Model file for the job. Use its own axes, mm. A direction names the side the tool comes from. Coordinates: 2 decimals unless noted, no trailing zeros. Order: outer loops, then holes, each group sorted by start corner. A loop starts at its lowest first (then second) coordinate and runs counter-clockwise, first axis right, second up. Notation, with made-up numbers: (-12, 13) - (8, 13) arc R27 cw to (8, 49) - close; hole circle Ø7 at (-21, 54). An arc over 180 degrees is marked (long way). Put each result on its own line as item: value. Start each with the question number.
Autodesk Fusion 360 part; units mm, degrees
sketch "Sketch1" plane through (0, 0, 0) normal (0, 0, 1) x (1, 0, 0)
  line L0 (0, 0) -> (60, 0)
  line L1 (60, 0) -> (60, -25)
  line L2 (60, -25) -> (0, -25)
  line L3 (0, -25) -> (0, 0)
  line L4 (5, -5) -> (55, -5)
  line L5 (55, -5) -> (55, -20)
  line L6 (55, -20) -> (5, -20)
  line L7 (5, -20) -> (5, -5)
  line L8 (41, -10.5) -> (45, -10.5)
  line L9 (45, -10.5) -> (45, -14.5)
  line L10 (45, -14.5) -> (41, -14.5)
  line L11 (41, -14.5) -> (41, -10.5)
  line L12 (15, -10.5) -> (19, -10.5)
  line L13 (19, -10.5) -> (19, -14.5)
  line L14 (19, -14.5) -> (15, -14.5)
  line L15 (15, -14.5) -> (15, -10.5)
  dimension "d1" = 60
  dimension "d2" = 25
  dimension "d3" = 50
  dimension "d4" = 15
  dimension "d5" = 5
  dimension "d6" = 5
  dimension "d7" = 4
  dimension "d8" = 10
  dimension "d9" = 5.5
  dimension "d10" = 4
  dimension "d11" = 4
  dimension "d12" = 5.5
  dimension "d13" = 10
  dimension "d14" = 4
extrude "Extrude1" add sketch "Sketch1" along normal blind 2 contours L0 L1 L2 L3
sketch "Sketch2" plane through (0, 0, 0) normal (0, 0, 1) x (1, 0, 0)
  line L0 (15, -10.5) -> (19, -10.5)
  line L1 (19, -10.5) -> (19, -14.5)
  line L2 (19, -14.5) -> (15, -14.5)
  line L3 (15, -14.5) -> (15, -10.5)
  line L4 (41, -10.5) -> (45, -10.5)
  line L5 (45, -10.5) -> (45, -14.5)
  line L6 (45, -14.5) -> (41, -14.5)
  line L7 (41, -14.5) -> (41, -10.5)
  line L8 (55, -5) -> (55, -20)
  line L9 (55, -20) -> (5, -20)
  line L10 (5, -20) -> (5, -5)
  line L11 (5, -5) -> (55, -5)
  dimension "d17" = 4
  dimension "d18" = 10
  dimension "d19" = 5.5
  dimension "d20" = 4
  dimension "d21" = 4
  dimension "d22" = 10
  dimension "d23" = 5.5
  dimension "d24" = 4
extrude "Extrude2" add sketch "Sketch2" along normal blind 5
extrude "Extrude3" add 1 faces at (40, -25, 0.6667) along direction (0, -1, 0) blind 10
extrude "Extrude4" add 1 faces at (20, 0, 0.6667) along direction (0, 1, 0) blind 10
sketch "Sketch3" plane through (0, -35, 0) normal (0, -1, 0) x (1, 0, 0)
  line L0 (0, 0) -> (60, 0)
  line L1 (60, 0) -> (60, 2)
  line L2 (60, 2) -> (0, 2)
  line L3 (0, 2) -> (0, 0)
  line L4 (25, 0) -> (35, 0)
  line L5 (35, 0) -> (35, 1)
  line L6 (35, 1) -> (25, 1)
  line L7 (25, 1) -> (25, 0)
  line L8 (41, 0) -> (41, 5)
  dimension "d31" = 1
  dimension "d32" = 6
  dimension "d33" = 10
extrude "Extrude5" add sketch "Sketch3" along normal blind 50 contours L0 L4 L5 L6 L7
sketch "Sketch4" plane through (0, 10, 0) normal (0, 1, 0) x (-1, 0, 0)
  line L0 (-60, 0) -> (0, 0)
  line L1 (0, 0) -> (0, 2)
  line L2 (0, 2) -> (-60, 2)
  line L3 (-60, 2) -> (-60, 0)
  line L4 (-35, 1) -> (-25, 1)
  line L5 (-25, 1) -> (-25, 0)
  line L6 (-25, 0) -> (-35, 0)
  line L7 (-35, 0) -> (-35, 1)
  line L8 (-19, 0) -> (-19, 5)
  line L9 (-41, 0) -> (-41, 5)
  dimension "d36" = 6
  dimension "d37" = 1
  dimension "d38" = 6
extrude "Extrude6" add sketch "Sketch4" along normal blind 50 contours L0 L4 L5 L6 L7
sketch "Sketch5" plane through (35, 0, 0) normal (1, 0, 0) x (0, 1, 0)
  line L0 (-35, 0) -> (-35, 1)
  line L1 (-35, 1) -> (-85, 1)
  line L2 (-85, 1) -> (-85, 0)
  line L3 (-85, 0) -> (-35, 0)
  line L4 (-85, 1) -> (-83, 1)
  line L5 (-83, 1) -> (-83, 0)
  line L6 (-83, 0) -> (-85, 0)
  line L7 (-85, 0) -> (-85, 1)
  dimension "d41" = 2
extrude "Extrude7" add sketch "Sketch5" along normal blind 25 contours L1 L2 L3 L4 L5 L6 L7
sketch "Sketch6" plane through (25, 0, 0) normal (-1, 0, 0) x (0, -1, 0)
  line L0 (35, 1) -> (35, 0)
  line L1 (35, 0) -> (85, 0)
  line L2 (85, 0) -> (85, 1)
  line L3 (85, 1) -> (35, 1)
  line L4 (85, 0) -> (83, 0)
  line L5 (83, 0) -> (83, 1)
  line L6 (83, 1) -> (85, 1)
  line L7 (85, 1) -> (85, 0)
  dimension "d44" = 2
extrude "Extrude8" add sketch "Sketch6" along normal blind 25 contours L1 L2 L3 L4 L5 L6 L7
sketch "Sketch7" plane through (25, 0, 0) normal (-1, 0, 0) x (0, -1, 0)
  line L0 (-10, 0) -> (-10, 1)
  line L1 (-10, 1) -> (-60, 1)
  line L2 (-60, 1) -> (-60, 0)
  line L3 (-60, 0) -> (-10, 0)
  line L4 (-60, 1) -> (-58, 1)
  line L5 (-58, 1) -> (-58, 0)
  line L6 (-58, 0) -> (-60, 0)
  line L7 (-60, 0) -> (-60, 1)
  dimension "d47" = 2
extrude "Extrude9" add sketch "Sketch7" along normal blind 25 contours L1 L2 L3 L4 L5 L6 L7
sketch "Sketch8" plane through (35, 0, 0) normal (1, 0, 0) x (0, 1, 0)
  line L0 (10, 1) -> (10, 0)
  line L1 (10, 0) -> (60, 0)
  line L2 (60, 0) -> (60, 1)
  line L3 (60, 1) -> (10, 1)
  line L4 (58, 1) -> (60, 1)
  line L5 (60, 1) -> (60, 0)
  line L6 (60, 0) -> (58, 0)
  line L7 (58, 0) -> (58, 1)
  dimension "d50" = 2
extrude "Extrude10" add sketch "Sketch8" along normal blind 25 contours L1 L2 L3 L4 L5 L6 L7
sketch "Sketch9" plane through (0, 0, 5) normal (0, 0, 1) x (-1, 0, 0)
  line L0 (-19, 14.5) -> (-15, 14.5)
  line L1 (-15, 14.5) -> (-15, 10.5)
  line L2 (-15, 10.5) -> (-19, 10.5)
  line L3 (-45, 14.5) -> (-41, 14.5)
  line L4 (-41, 14.5) -> (-41, 10.5)
  line L5 (-41, 10.5) -> (-45, 10.5)
  line L6 (-45, 10.5) -> (-45, 14.5)
  line L7 (-5, 5) -> (-5, 20)
  line L8 (-5, 20) -> (-55, 20)
  line L9 (-55, 20) -> (-55, 5)
  line L10 (-55, 5) -> (-5, 5)
Item 1: Slice it at C-C, the plane x = 43. Give the cut face in (y, z), plus the area to 3 significant figures.
Item 2: Flat gauge pins, fed straight in: pin 1 Ø25 at (x, y) = (27, 34.5) entering from +Z; pin 2 Ø1.5 at (y, z) = (-14.5, 3.5) entering from -X; pin 3 Ø0.5 at (y, z) = (41.5, 0.5) entering from -X. Where does each tip first touch, or does it go through?
Item 3: Wall check: line 1 along Y through (x, z) = (22, 3.55); line 2 along X through (y, z) = (-76.5, 0.25); line 3 along Z through (x, y) = (16, 0.5). Give the ranges that are in metal, low to high.
Item 4: 3-axis set-ups, long thin cutter, end or side, ignore diameter. For faces 4 (the face through (55, -12, 3)), 5 (the face through (41, -13, 2)), 6 (the face through (30, 37, 1)): which of +Z, -Z, +X, -X, +Y, -Y reach the whole face in a straight line?
Item 5: Slice it at D-D, the plane y = -49. Give the cut face in (x, z).
Item 6: Pull direction X, two halves, no side cores. Call faces 1 (the face through (30, -62, 1)), 2 (the face through (5, -13, 3)), 3 (the face through (19, -12, 2)): pulls with the +X half, pulls with the -X half, needs draft (parallel to the pull), parting line crosses it, or undercut.
Item 7: Slice it at A-A, the plane x = 13. Give the cut face in (y, z), plus the area to 3 significant figures.
Item 8: Slice it at B-B, the plane z = 2.9. Give the cut face in (x, y), plus the area to 3 significant figures.
Here are the results:
1. outline: (-85, 0) - (-83, 0) - (-83, 1) - (-85, 1) - close; (-35, 0) - (-14.5, 0) - (-14.5, 5) - (-20, 5) - (-20, 2) - (-35, 2) - close; (-10.5, 0) - (10, 0) - (10, 2) - (-5, 2) - (-5, 5) - (-10.5, 5) - close; (58, 0) - (60, 0) - (60, 1) - (58, 1) - close
1. area: 119 mm^2
2. pin 1: stops at z = 1
2. pin 2: stops at x = 5
2. pin 3: stops at x = 25
3. line 1: y = -20 to -5
3. line 2: x = 25 to 35
3. line 3: z = 0 to 2
4. face 4: +Z, +X, +Y, -Y
4. face 5: +Z, -Z
4. face 6: +Z, +X, -X, +Y
5. outline: (25, 0) - (35, 0) - (35, 1) - (25, 1) - close
6. face 1: needs draft
6. face 2: pulls with the -X half
6. face 3: undercut
7. outline: (-85, 0) - (-83, 0) - (-83, 1) - (-85, 1) - close; (-35, 0) - (10, 0) - (10, 2) - (-5, 2) - (-5, 5) - (-20, 5) - (-20, 2) - (-35, 2) - close; (58, 0) - (60, 0) - (60, 1) - (58, 1) - close
7. area: 139 mm^2
8. outline: (5, -20) - (55, -20) - (55, -5) - (5, -5) - close; hole (15, -14.5) - (19, -14.5) - (19, -10.5) - (15, -10.5) - close; hole (41, -14.5) - (45, -14.5) - (45, -10.5) - (41, -10.5) - close
8. area: 718 mm^2
